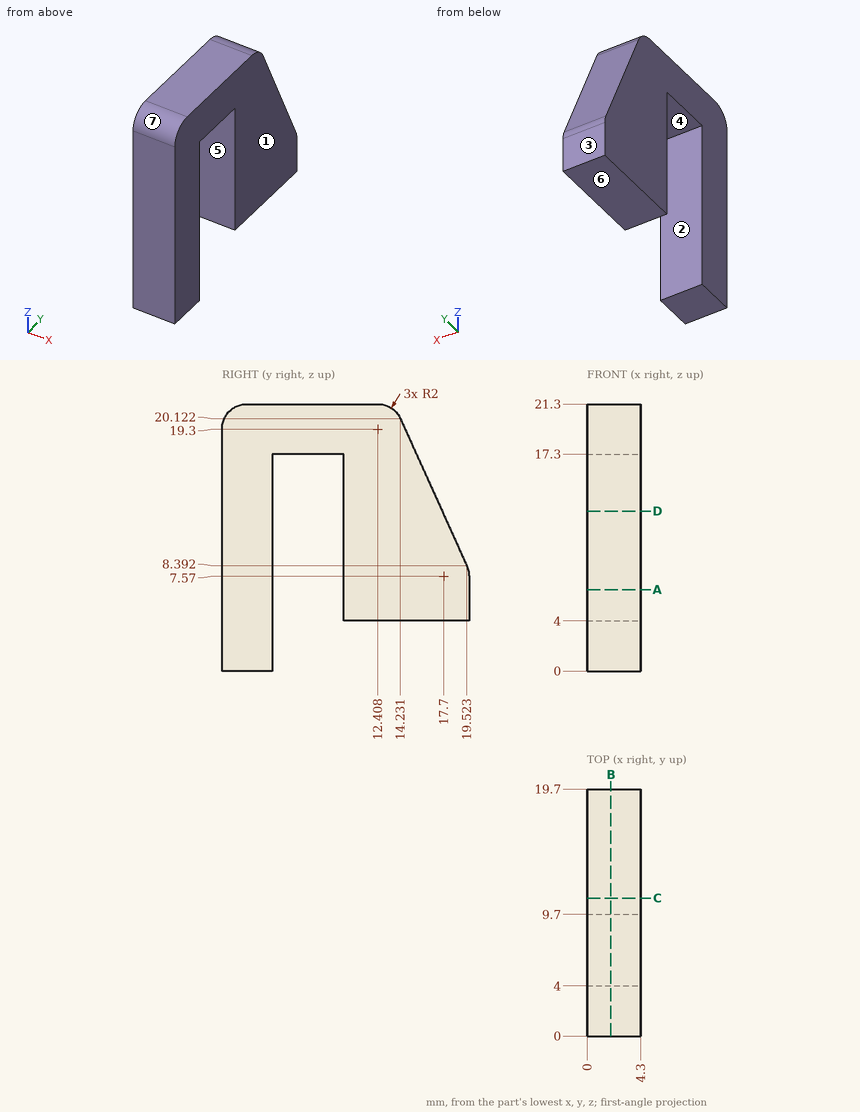
Geometry check sheet. Reference: drawing and pictorial views, mm from the part's lowest x, y, z. A direction names the side the tool comes from. Round coordinates to 2 decimals unless told otherwise and drop trailing zeros. Order: outer loops, then holes, each group sorted by start corner. A loop starts at its lowest first (then second) coordinate and runs counter-clockwise, first axis right, second up. Notation, with made-up numbers: (0.25, 76) - (10.25, 76) arc R22 ccw to (10.25, 106) - close; hole circle Ø1 at (39.5, 18). An arc over 180 degrees is marked (long way). Use a Markdown table: item, result. Add a question column.
1) Section check B-B (x = 1.9). Record the cut outline in (y, z), then the cut area to 3 significant figures.
2) Set-up check for the marked faces 5, 6 and 7: record each of +Z, -Z, +X, -X, +Y, -Y from which the full face is reachable in a straight line by a thin tool's end or side.
3) Section check C-C (y = 11). Record the cut outline in (x, z), then the cut area to 3 significant figures.
4) Thickness scan on line 1 along Y through (x, z) = (2.35, 5); line 2 along Z through (x, y) = (1.4, 9); line 3 along Y through (x, z) = (1.9, 16.25). Record the ranges inside material, lowest first.
5) Section check A-A (z = 6.5). Record the cut outline in (x, y).
6) Section check D-D (z = 12.75). Record the cut outline in (x, y).
7) Gauge pin test, flat ends, axial feed: P1, Ø2, axis at x = 3, z = 15.5, coming from the -Y side; P2, Ø1.3, axis at x = 3, z = 11, coming from the +Y side; P3, Ø2, axis at x = 1, z = 16.5, coming from the +Y side; P4, Ø1.3, axis at x = 2, y = 12.5, coming from the -Z side. Record the tip position at first contact, or that the pin passes through.
8) Mould release check, pull along Y, two halves, no side actions. Record for the marked faces 1, 2, 3 and 4: released by +Y, released by -Y, zero draft, split by the parting line, or undercut.
Established:
| question | item | result |
|---|---|---|
| 1 | outline | (0, 0) - (4, 0) - (4, 17.3) - (9.7, 17.3) - (9.7, 4) - (19.7, 4) - (19.7, 7.57) arc R2 ccw to (19.52, 8.39) - (14.23, 20.12) arc R2 ccw to (12.41, 21.3) - (2, 21.3) arc R2 ccw to (0, 19.3) - close |
| 1 | area | 240 mm2 |
| 2 | face 5 | -Z, +X, -X |
| 2 | face 6 | -Z, +X, -X, +Y |
| 2 | face 7 | +Z, +X, -X, -Y |
| 3 | outline | (0, 4) - (4.3, 4) - (4.3, 21.3) - (0, 21.3) - close |
| 3 | area | 74.4 mm2 |
| 4 | line 1 | 0 to 4, 9.7 to 19.7 |
| 4 | line 2 | 17.3 to 21.3 |
| 4 | line 3 | 0 to 4, 9.7 to 15.98 |
| 5 | outline | (0, 0) - (4.3, 0) - (4.3, 4) - (0, 4) - close; (0, 9.7) - (4.3, 9.7) - (4.3, 19.7) - (0, 19.7) - close |
| 6 | outline | (0, 0) - (4.3, 0) - (4.3, 4) - (0, 4) - close; (0, 9.7) - (4.3, 9.7) - (4.3, 17.56) - (0, 17.56) - close |
| 7 | P1 | y = 0 |
| 7 | P2 | y = 18.64 |
| 7 | P3 | y = 16.32 |
| 7 | P4 | z = 4 |
| 8 | face 1 | zero draft |
| 8 | face 2 | undercut |
| 8 | face 3 | released by +Y |
| 8 | face 4 | undercut |
